Input: part model. Units: mm. Frame: model coordinates. A direction names the side the tool comes from. Round coordinates to 2 decimals unless told otherwise and drop trailing zeros. Order: outer loops, then holes, each group sorted by start corner. A loop starts at its lowest first (then second) coordinate and runs counter-clockwise, first axis right, second up. Notation, with made-up numbers: (10, 28) -> (16, 28) arc R31 cw to (16, 56) -> close; hole circle Ø6 at (-0.5, 77). An arc over 180 degrees is marked (long way). Answer as CSV lines item,"result". Start each with the question number.
1) First-contact query: P1, Ø4, axis at x = 7.5, y = -10.5, coming from the -Z side. Flat tip, straight axial feed; report the tip coordinate or a pass-through.
2) Section query D-D, the plane y = -11.5. Output: boundary loops of the cut face in (x, z), and give its area (3 significant figures).
3) Access query for faces 1 (the face through (1, -16.563, -1)), 2 (the face through (-15.263, 12.582, -0.732)). Directions: +Z, -Z, +X, -X, +Y, -Y. A direction counts if a zero-diameter tool reaches every point of the face in a straight line with its end or side. Return the directions, or none.
4) Section query C-C, the plane z = -1.55. Output: boundary loops of the cut face in (x, y), and give its area (3 significant figures).
5) Line query: L1, parallel to Y at x = -3, z = 0.3; L2, parallel to Y at x = -7.5, z = -0.4; L3, parallel to X at y = -13.5, z = -1.1. Output: solid intervals per line, ascending.
6) Section query B-B, the plane x = -3. Output: boundary loops of the cut face in (y, z).
7) Mould query, pull axis Y, two halves, no side actions, for faces 3 (the face through (-14.165, -3, -1)), 4 (the face through (-16.165, -4, -1)), 5 (the face through (14.835, -3, -1)), 6 (the face through (15.98, 12.535, -0.732)). Classes: +Y half, -Y half, draft (parallel to the pull), parting line (faces both ways), or undercut.
8) Section query A-A, the plane y = 2.5. Output: boundary loops of the cut face in (x, z), and give its area (3 significant figures).
```python
from build123d import *

# Parameters (mm, degrees)
SKETCH_1_W      = 33
SKETCH_1_H      = 32
SKETCH_1_W_2    = 26
SKETCH_1_H_2    = 16.1
EXTRUDE_1_DEPTH = 0.5
SKETCH_2_W      = 33
SKETCH_2_H      = 32
SKETCH_2_W_2    = 29
SKETCH_2_H_2    = 28
EXTRUDE_2_DEPTH = 2
FILLET_1_R      = 3
FILLET_2_R      = 3


with BuildPart() as part:
    # 草图1 → 凸台-拉伸1 (new body)
    with BuildSketch(Plane.XY):
        with Locations((0.334983498, -2.562706271)):
            Rectangle(SKETCH_1_W, SKETCH_1_H)
        with Locations((0.334983498, -1.212706271)):
            Rectangle(SKETCH_1_W_2, SKETCH_1_H_2, mode=Mode.SUBTRACT)
    extrude(amount=EXTRUDE_1_DEPTH)

    # 草图2 → 凸台-拉伸2 (add)
    with BuildSketch(Plane(origin=(0, 0, 0), x_dir=(-1, 0, 0), z_dir=(0, 0, -1))):
        with Locations((-0.334983498, -2.562706271)):
            Rectangle(SKETCH_2_W, SKETCH_2_H)
        with Locations((-0.334983498, -2.562706271)):
            Rectangle(SKETCH_2_W_2, SKETCH_2_H_2, mode=Mode.SUBTRACT)
    extrude(amount=EXTRUDE_2_DEPTH)

    # 圆角1
    fillet_1_edges = [part.edges().sort_by_distance(p)[0] for p in [
        (16.834983498, 13.437293729, -0.75),
    ]]
    fillet(fillet_1_edges, radius=FILLET_1_R)

    # 圆角2
    fillet_2_edges = [part.edges().sort_by_distance(p)[0] for p in [
        (-16.165016502, 13.437293729, -0.75),
    ]]
    fillet(fillet_2_edges, radius=FILLET_2_R)


solid = part.part
```
Findings:
1,P1,"stops at z = 0"
2,outline,"(-16.17, -2) -> (-14.17, -2) -> (-14.17, 0) -> (14.83, 0) -> (14.83, -2) -> (16.83, -2) -> (16.83, 0.5) -> (-16.17, 0.5) -> close"
2,area,"24.5 mm^2"
3,face 1,"-Z"
3,face 2,"+Z, -Z, -X, +Y"
4,outline,"(-16.17, -18.56) -> (16.83, -18.56) -> (16.83, 10.44) arc R3 ccw to (13.83, 13.44) -> (-13.17, 13.44) arc R3 ccw to (-16.17, 10.44) -> close; hole (-14.17, -16.56) -> (14.83, -16.56) -> (14.83, 11.44) -> (-14.17, 11.44) -> close"
4,area,"240 mm^2"
5,L1,"y = -18.56 to -9.26, 6.84 to 13.44"
5,L2,"y = -18.56 to -16.56, 11.44 to 13.44"
5,L3,"x = -16.17 to -14.17, 14.83 to 16.83"
6,outline,"(-18.56, -2) -> (-16.56, -2) -> (-16.56, 0) -> (-9.26, 0) -> (-9.26, 0.5) -> (-18.56, 0.5) -> close; (6.84, 0) -> (11.44, 0) -> (11.44, -2) -> (13.44, -2) -> (13.44, 0.5) -> (6.84, 0.5) -> close"
7,face 3,"undercut"
7,face 4,"draft"
7,face 5,"undercut"
7,face 6,"+Y half"
8,outline,"(-16.17, -2) -> (-14.17, -2) -> (-14.17, 0) -> (-12.67, 0) -> (-12.67, 0.5) -> (-16.17, 0.5) -> close; (13.33, 0) -> (14.83, 0) -> (14.83, -2) -> (16.83, -2) -> (16.83, 0.5) -> (13.33, 0.5) -> close"
8,area,"11.5 mm^2"
